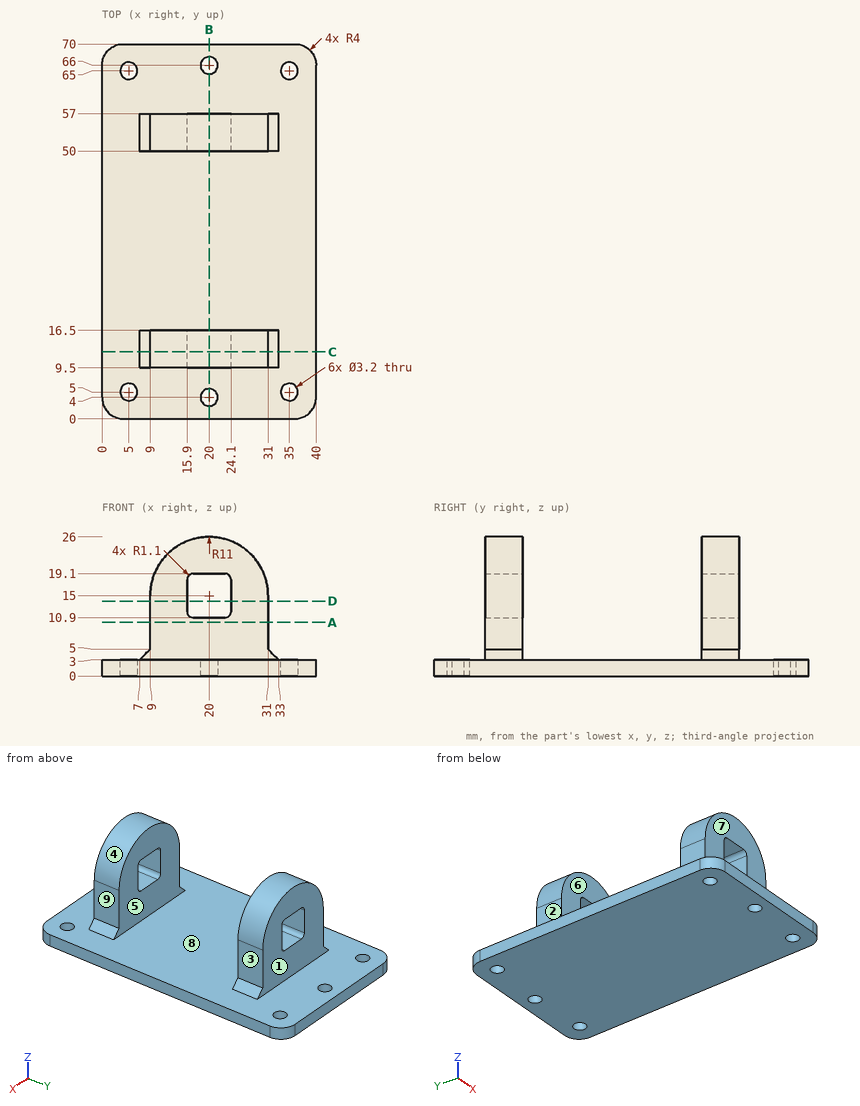
Verification items for this drawing (mm, ordinates from the low corner). A direction names the side the tool comes from. Give positions to 0.01 mm unless a question says otherwise; leave off trailing zeros. Loops run counter-clockwise (first coordinate to the right, second up) from the corner with the lowest first, then second, coordinate; pieces in that order, holes last. Notation, with made-up numbers: M 33,46.5 L 76,46.5 A20 ccw 76,68.5 Z; hole C 5,-6.5 d9. An arc over 180 degrees is marked long. Answer in a Markdown table with one row per item.
1) Mould release check, pull along Y, two halves, no side actions. Record for the marked faces 6, 7, 8 and 9: released by +Y, released by -Y, zero draft, split by the parting line, or undercut.
Solutions:
| item | result |
|---|---|
| face 6 | undercut |
| face 7 | released by -Y |
| face 8 | undercut |
| face 9 | zero draft |
2) Cross-section at A-A (z = 10). Enter the section's corners in (x, y).
Solutions:
| item | result |
|---|---|
| outline | M 9,9.5 L 31,9.5 L 31,16.5 L 9,16.5 Z; M 9,50 L 31,50 L 31,57 L 9,57 Z |
3) Depth check by flat-ended pin: pin 1 (6 mm diameter, centred on x = 10.5, z = 7, fed in from -Y); pin 2 (1.8 mm diameter, centred on y = 11.5, z = 13.5, fed in from -X); pin 3 (12 mm diameter, centred on x = 5, y = 8, fed in from +Z). Enter the tip coordinate at first touch or a pass-through.
Solutions:
| item | result |
|---|---|
| pin 1 | stops at y = 9.5 |
| pin 2 | stops at x = 9 |
| pin 3 | stops at z = 21.04 |
4) Tool access check on the marked faces 1, 2, 3, 4 and 5. Record the directions out of +Z, -Z, +X, -X, +Y, -Y that give a thin tool (end or side, any length) a straight path to the whole face; none if there is none.
Solutions:
| item | result |
|---|---|
| face 1 | +Z, +X, -X, +Y |
| face 2 | +Z, -X, +Y, -Y |
| face 3 | +Z, +X, +Y, -Y |
| face 4 | +Z, +Y, -Y |
| face 5 | +Z, +X, -X |
5) Cross-section at B-B (x = 20). Enter the section's corners in (y, z).
Solutions:
| item | result |
|---|---|
| outline | M 0,0 L 2.4,0 L 2.4,3 L 0,3 Z; M 5.6,0 L 64.4,0 L 64.4,3 L 57,3 L 57,10.9 L 50,10.9 L 50,3 L 16.5,3 L 16.5,10.9 L 9.5,10.9 L 9.5,3 L 5.6,3 Z; M 9.5,19.1 L 16.5,19.1 L 16.5,26 L 9.5,26 Z; M 50,19.1 L 57,19.1 L 57,26 L 50,26 Z; M 67.6,0 L 70,0 L 70,3 L 67.6,3 Z |
6) Thickness scan on line 1 (Y direction, x = 5, z = 1.85); line 2 (Y direction, x = 20, z = 1.8); line 3 (Y direction, x = 16, z = 20.25). Record the ranges inside material, lowest first.
Solutions:
| item | result |
|---|---|
| line 1 | y = 0 to 3.4, 6.6 to 63.4, 66.6 to 70 |
| line 2 | y = 0 to 2.4, 5.6 to 64.4, 67.6 to 70 |
| line 3 | y = 9.5 to 16.5, 50 to 57 |
7) Cross-section at D-D (z = 14). Enter the section's corners in (x, y), plus the area to 3 significant figures.
Solutions:
| item | result |
|---|---|
| outline | M 9,9.5 L 15.9,9.5 L 15.9,16.5 L 9,16.5 Z; M 9,50 L 15.9,50 L 15.9,57 L 9,57 Z; M 24.1,9.5 L 31,9.5 L 31,16.5 L 24.1,16.5 Z; M 24.1,50 L 31,50 L 31,57 L 24.1,57 Z |
| area | 193 mm^2 |
8) Cross-section at C-C (y = 12.5). Enter the section's corners in (x, z).
Solutions:
| item | result |
|---|---|
| outline | M 0,0 L 40,0 L 40,3 L 33,3 L 31,5 L 31,15 A11 ccw 9,15 L 9,5 L 7,3 L 0,3 Z; hole M 15.9,12 A1.1 ccw 17,10.9 L 23,10.9 A1.1 ccw 24.1,12 L 24.1,18 A1.1 ccw 23,19.1 L 17,19.1 A1.1 ccw 15.9,18 Z |
